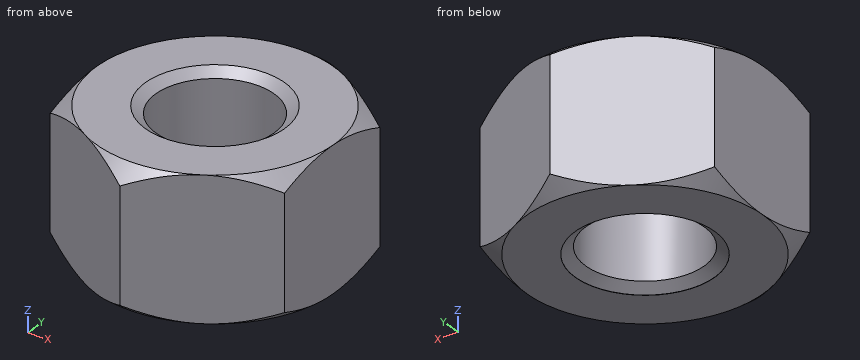
from build123d import *

# Parameters (mm, degrees)
BASENUT_START = -16.0274
BASENUTSKE_R  = 6.74624
BASENUT_DEPTH = 16.0274


with BuildPart() as part:
    # BaseNutSke → BaseNut (new body)
    with BuildSketch(Plane.XY.offset(BASENUT_START)):
        Polygon((13.4874, 7.786954021), (13.4874, -7.786954021), (0, -15.573908041), (-13.4874, -7.786954021), (-13.4874, 7.786954021), (0, 15.573908041), align=None)
        Circle(BASENUTSKE_R, mode=Mode.SUBTRACT)
    extrude(amount=BASENUT_DEPTH)

    # Sketch3 → Double-Chamfer (revolve, cut)
    with BuildSketch(Plane(origin=(0, 0, 0), x_dir=(0, 0, -1), z_dir=(1, 0, 0))):
        Polygon((16.0274, 13.4874), (14.4399, 15.573908041), (14.4399, 28.273908041), (28.7274, 28.273908041), (28.7274, 13.4874), align=None)
        Polygon((1.5875, 28.273908041), (-12.7, 28.273908041), (-12.7, 13.4874), (0, 13.4874), (1.5875, 15.573908041), align=None)
    revolve(axis=Axis((0, 0, 0), (0, 0, -1)), mode=Mode.SUBTRACT)

    # Sketch5 → EndChamfer (revolve, cut)
    with BuildSketch(Plane(origin=(0, 0, 0), x_dir=(0, 0, -1), z_dir=(1, 0, 0)), mode=Mode.PRIVATE) as endchamfer_sk:
        Polygon((16.002, 7.9375), (15.084457845, 6.627114), (16.0528, 6.627114), (16.0528, 7.9375), align=None)
        Polygon((-0.0508, 7.9375), (0, 7.9375), (0.917542155, 6.627114), (-0.0508, 6.627114), align=None)
    revolve(endchamfer_sk.sketch.rotate(Axis((0, 0, -25.037505729), (0, 0, -1)), 90), axis=Axis((0, 0, -25.037505729), (0, 0, -1)), mode=Mode.SUBTRACT)


solid = part.part
Geometry: final body of the model. Coordinates: model frame, mm. Round coordinates to 2 decimals unless told otherwise and drop trailing zeros. Order: outer loops, then holes, each group sorted by start corner. A loop starts at its lowest first (then second) coordinate and runs counter-clockwise, first axis right, second up.
Q1. Pin query (flat end, axial travel): pin 1 (15.5 mm diameter, centred on x = 0, y = 0, fed in from -Z); pin 2 (1 mm diameter, centred on x = -7, z = -13.5, fed in from -Y). Return the tip coordinate at first contact, or that it passes through.
Result sheet:
pin 1: stops at z = -15.87
pin 2: stops at y = -11.82
Q2. Section A-A, the plane z = -5.25. Output: boundary loops of the cut face in (x, y), and give its area (3 significant figures).
Result sheet:
outline: (-13.49, -7.79) - (0, -15.57) - (13.49, -7.79) - (13.49, 7.79) - (0, 15.57) - (-13.49, 7.79) - close; hole circle Ø13.49 at (0, 0)
area: 487 mm2
Q3. Material intervals for probe 1 along Y at (x, z) = (-1.5, -1.75); probe 2 along Y at (x, z) = (0, -15.95); probe 3 along Y at (x, z) = (7, -12), sorted ascending.
Result sheet:
probe 1: y = -14.71 to -6.58, 6.58 to 14.71
probe 2: y = -13.59 to -7.86, 7.86 to 13.59
probe 3: y = -11.53 to 11.53
